from build123d import *

# Parameters (mm, degrees)
F0_R     = 2.5
F1_DEPTH = 4.5
F2_DEPTH = 20
F3_W     = 3.25
F3_H     = 20
F4_DEPTH = 25
F5_R     = 1.5
F6_R     = 5


with BuildPart() as f1:
    # F0 (on Right) → F1 (new body, symmetric)
    with BuildSketch(Plane.YZ):
        with BuildLine():
            Line((-7.5, 9), (-7.5, 0))
            ThreePointArc((-7.5, 0), (0, -7.5), (7.5, 0))
            Line((7.5, 0), (7.5, 9))
            Line((7.5, 9), (-7.5, 9))
        make_face()
        Circle(F0_R, mode=Mode.SUBTRACT)
        Polygon((-20, 9), (-7.5, 9), (7.5, 9), (20, 9), (20, 11.5), (-20, 11.5), align=None)
    extrude(amount=F1_DEPTH, both=True)

    # F0 (on Right) → F2 (join, symmetric)
    with BuildSketch(Plane.YZ):
        Polygon((-20, 9), (-7.5, 9), (7.5, 9), (20, 9), (20, 11.5), (-20, 11.5), align=None)
    extrude(amount=F2_DEPTH, both=True)

    # F3 (on face) → F4 (cut)
    with BuildSketch(Plane(origin=(0, 0, 9), x_dir=(1, 0, 0), z_dir=(0, 0, -1))):
        Rectangle(F3_W, F3_H)
    extrude(amount=F4_DEPTH, mode=Mode.SUBTRACT)

    # F5
    f5_edges = [f1.edges().sort_by_distance(p)[0] for p in [
        (-4.5, 0, 9),
        (4.5, 0, 9),
        (-3.0625, 7.5, 9),
        (3.0625, 7.5, 9),
        (-3.0625, -7.5, 9),
        (3.0625, -7.5, 9),
    ]]
    fillet(f5_edges, radius=F5_R)

    # F6
    f6_edges = [f1.edges().sort_by_distance(p)[0] for p in [
        (20, -20, 10.25),
        (-20, -20, 10.25),
        (20, 20, 10.25),
        (-20, 20, 10.25),
    ]]
    fillet(f6_edges, radius=F6_R)


solid = f1.part
The listing builds one solid part. Answer for the finished solid, in the listing's coordinates (mm). A direction names the side the tool comes from. Round coordinates to 2 decimals unless told otherwise and drop trailing zeros. Write each loop counter-clockwise with the first axis right and the second up, starting at its lowest first coordinate (ties: lowest second). Pieces come first, ordered by that corner, then holes. Notation, with made-up numbers: (-22.75, 38) - (-16.75, 38) arc R30 cw to (-16.75, 77) - close; hole circle Ø6 at (64.5, 62). An arc over 180 degrees is marked (long way). Use a Markdown table: item, result. Add a question column.
1. The part is cut by section A-A (y = 0). Write down the section's boundary in (x, z) (3 decimals).
2. A tool of negligible diameter and unlimited length cuts with its end or side. For faces 4 (the face through (-4.5, -2, 2)), 5 (the face through (4.5, -2, 2)), 6 (the face through (-1.625, 0, 3)), from which of +Z, -Z, +X, -X, +Y, -Y can it reach the whole face along a straight path? Write none if from no direction.
3. Consider line 1 (X direction, y = -5.5, z = 1.5) (3 decimals); line 2 (Z direction, x = 2, y = 0); line 3 (Y direction, x = -3.7, z = 0). Determine where each line is inside the solid, lowest interval first.
4. The part is cut by section C-C (z = 1.25). Write down the section's boundary in (x, y) (3 decimals).
5. The part is cut by section B-B (z = -4.5). Write down the section's boundary in (x, y) (3 decimals).
6. For a pull along Z with two mould halves and no side action, classify faces 1 (the face through (3.04, -0.54, -2.44)), 2 (the face through (-3.36, -7.95, 8.57)), 3 (the face through (3, 7.5, 4)) as +Z half, -Z half, draft (parallel to the pull), parting line (faces both ways), or undercut.
7. Flat-ended cylindrical pins translate along their axes: P1, Ø6.5, axis at y = 0, z = 0, coming from the -X side; P2, Ø10, axis at x = 11.5, z = -5, coming from the +Y side; P3, Ø8, axis at y = 0, z = 0, coming from the +X side; P4, Ø0.9, axis at x = -3, z = 4.5, coming from the -Y side. Find the tip coordinate at first contact, or state that the pin passes through.
8. The part is cut by section D-D (x = 13.5). Write down the section's boundary in (y, z), and give its area (3 significant figures).
Reported:
| question | item | result |
|---|---|---|
| 1 | outline | (-20, 9) - (-6, 9) arc R1.5 cw to (-4.5, 7.5) - (-4.5, 2.5) - (-1.625, 2.5) - (-1.625, 9) - (1.625, 9) - (1.625, 2.5) - (4.5, 2.5) - (4.5, 7.5) arc R1.5 cw to (6, 9) - (20, 9) - (20, 11.5) - (-20, 11.5) - close; (-4.5, -7.5) - (-1.625, -7.5) - (-1.625, -2.5) - (-4.5, -2.5) - close; (1.625, -7.5) - (4.5, -7.5) - (4.5, -2.5) - (1.625, -2.5) - close |
| 2 | face 4 | -Z, -X, +Y, -Y |
| 2 | face 5 | -Z, +X, +Y, -Y |
| 2 | face 6 | -Z, +Y, -Y |
| 3 | line 1 | -4.5 to -1.625, 1.625 to 4.5 |
| 3 | line 2 | -7.5 to -2.5, 2.5 to 11.5 |
| 3 | line 3 | -7.5 to -2.5, 2.5 to 7.5 |
| 4 | outline | (-4.5, -7.5) - (-1.625, -7.5) - (-1.625, -2.165) - (-4.5, -2.165) - close; (-4.5, 2.165) - (-1.625, 2.165) - (-1.625, 7.5) - (-4.5, 7.5) - close; (1.625, -7.5) - (4.5, -7.5) - (4.5, -2.165) - (1.625, -2.165) - close; (1.625, 2.165) - (4.5, 2.165) - (4.5, 7.5) - (1.625, 7.5) - close |
| 5 | outline | (-4.5, -6) - (-1.625, -6) - (-1.625, 6) - (-4.5, 6) - close; (1.625, -6) - (4.5, -6) - (4.5, 6) - (1.625, 6) - close |
| 6 | face 1 | undercut |
| 6 | face 2 | -Z half |
| 6 | face 3 | draft |
| 7 | P1 | x = -4.5 |
| 7 | P2 | through |
| 7 | P3 | x = 4.5 |
| 7 | P4 | y = -7.5 |
| 8 | outline | (-20, 9) - (20, 9) - (20, 11.5) - (-20, 11.5) - close |
| 8 | area | 100 mm^2 |
